Autodesk Inventor part; units mm, degrees
ref_plane "C1_XY" through (0, 0, 0) normal (0, 0, 1) x (1, 0, 0)
ref_plane "C1_YZ" through (0, 0, 0) normal (1, 0, 0) x (0, 1, 0)
ref_plane "C1_ZX" through (0, 0, 0) normal (0, 1, 0) x (0, 0, 1)
sketch "Sketch_1" plane through (0, 0, 0) normal (0, 0, 1) x (1, 0, 0)
  line L0 (-15, -4) -> (-15, -13)
  arc A0 (-15, -13) -> (-13, -15) centre (-13, -13) ccw
  line L1 (-13, -15) -> (-4, -15)
  line L2 (-4, -15) -> (-4, -13)
  line L3 (-4, -13) -> (-8.25, -13)
  line L4 (-8.25, -13) -> (-8.25, -9.6642)
  line L5 (-8.25, -9.6642) -> (-4.5858, -6)
  line L6 (-4.5858, -6) -> (-0.5196, -6)
  line L7 (-0.5196, -6) -> (0, -5.7)
  line L8 (0, -5.7) -> (0.5196, -6)
  line L9 (0.5196, -6) -> (4.5858, -6)
  line L10 (4.5858, -6) -> (8.25, -9.6642)
  line L11 (8.25, -9.6642) -> (8.25, -13)
  line L12 (8.25, -13) -> (4, -13)
  line L13 (4, -13) -> (4, -15)
  line L14 (4, -15) -> (13, -15)
  arc A1 (13, -15) -> (15, -13) centre (13, -13) ccw
  line L15 (15, -13) -> (15, -4)
  line L16 (15, -4) -> (13, -4)
  line L17 (13, -4) -> (13, -8.25)
  line L18 (13, -8.25) -> (9.6642, -8.25)
  line L19 (9.6642, -8.25) -> (6, -4.5858)
  line L20 (6, -4.5858) -> (6, -0.5196)
  line L21 (6, -0.5196) -> (5.7, 0)
  line L22 (5.7, 0) -> (6, 0.5196)
  line L23 (6, 0.5196) -> (6, 4.5858)
  line L24 (6, 4.5858) -> (9.6642, 8.25)
  line L25 (9.6642, 8.25) -> (13, 8.25)
  line L26 (13, 8.25) -> (13, 4)
  line L27 (13, 4) -> (15, 4)
  line L28 (15, 4) -> (15, 13)
  arc A2 (15, 13) -> (13, 15) centre (13, 13) ccw
  line L29 (13, 15) -> (4, 15)
  line L30 (4, 15) -> (4, 13)
  line L31 (4, 13) -> (8.25, 13)
  line L32 (8.25, 13) -> (8.25, 9.6642)
  line L33 (8.25, 9.6642) -> (4.5858, 6)
  line L34 (4.5858, 6) -> (0.5196, 6)
  line L35 (0.5196, 6) -> (0, 5.7)
  line L36 (0, 5.7) -> (-0.5196, 6)
  line L37 (-0.5196, 6) -> (-4.5858, 6)
  line L38 (-4.5858, 6) -> (-8.25, 9.6642)
  line L39 (-8.25, 9.6642) -> (-8.25, 13)
  line L40 (-8.25, 13) -> (-4, 13)
  line L41 (-4, 13) -> (-4, 15)
  line L42 (-4, 15) -> (-13, 15)
  arc A3 (-13, 15) -> (-15, 13) centre (-13, 13) ccw
  line L43 (-15, 13) -> (-15, 4)
  line L44 (-15, 4) -> (-13, 4)
  line L45 (-13, 4) -> (-13, 8.25)
  line L46 (-13, 8.25) -> (-9.6642, 8.25)
  line L47 (-9.6642, 8.25) -> (-6, 4.5858)
  line L48 (-6, 4.5858) -> (-6, 0.5196)
  line L49 (-6, 0.5196) -> (-5.7, 0)
  line L50 (-5.7, 0) -> (-6, -0.5196)
  line L51 (-6, -0.5196) -> (-6, -4.5858)
  line L52 (-6, -4.5858) -> (-9.6642, -8.25)
  line L53 (-9.6642, -8.25) -> (-13, -8.25)
  line L54 (-13, -8.25) -> (-13, -4)
  line L55 (-13, -4) -> (-15, -4)
extrude "Extrusion1" add sketch "Sketch_1" against normal blind 586
sketch "Sketch2" plane through (0, 0, -586) normal (0, 0, -1) x (-1, 0, 0)
  point P0 (0, 0)
hole "Hole1" at (0, 0, -586) direction (0, 0, 1) diameter 6.8 depth 586
sketch "Sketch3" plane through (0, 0, -586) normal (0, 0, -1) x (-1, 0, 0)
  point P0 (-11.6, 11.6)
hole "Hole2" at (11.6, 11.6, -586) direction (0, 0, 1) diameter 4.2 depth 586
pattern_linear "Rectangular Pattern1" count 2 spacing 23.2 along (-1, 0, 0) count 2 spacing 23.2 along (0, -1, 0) of "Hole2"
sketch "Sketch_41" plane through (0, 0, 0) normal (1, 0, 0) x (0, 0, -1)
  line L0 (10, 0) -> (0.05, 0)
  line L1 (0.05, 2.5) -> (0.483, 2.067)
  line L2 (0.483, 2.067) -> (10, 2.067)
  line L3 (10, 2.067) -> (10, 3.45)
  line L4 (10, 3.45) -> (0.05, 3.45)
  line L5 (0.05, 3.45) -> (0.05, 2.5)
revolve "Revolution1" add sketch "Sketch_41" angle 360 about axis through (0, 0, -10) along (0, 0, -1)
thread "Thread1"
sketch "Sketch_42" plane through (0, 0, 0) normal (1, 0, 0) x (0, 0, -1)
  line L0 (585.95, 0) -> (576, 0)
  line L1 (576, 3.45) -> (576, 2.067)
  line L2 (576, 2.067) -> (585.517, 2.067)
  line L3 (585.517, 2.067) -> (585.95, 2.5)
  line L4 (585.95, 2.5) -> (585.95, 3.45)
  line L5 (585.95, 3.45) -> (576, 3.45)
revolve "Revolution2" add sketch "Sketch_42" angle 360 about axis through (0, 0, -585.95) along (0, 0, -1)
thread "Thread2"
ref_plane "C1_XY" through (0, 0, 0) normal (0, 0, 1) x (1, 0, 0)
ref_plane "C1_YZ" through (0, 0, 0) normal (1, 0, 0) x (0, 1, 0)
ref_plane "C1_ZX" through (0, 0, 0) normal (0, 1, 0) x (0, 0, 1)
ref_plane "to_frame_cap1_XY" through (0, 0, 0) normal (0, 0, 1) x (1, 0, 0)
ref_plane "to_frame_cap1_YZ" through (0, 0, 0) normal (1, 0, 0) x (0, 1, 0)
ref_plane "to_frame_cap1_ZX" through (0, 0, 0) normal (0, 1, 0) x (0, 0, 1)
ref_plane "to_frame_cap2_XY" through (0, 0, -586) normal (0, 0, -1) x (1, 0, 0)
ref_plane "to_frame_cap2_YZ" through (0, 0, -586) normal (1, 0, 0) x (0, -1, 0)
ref_plane "to_frame_cap2_ZX" through (0, 0, -586) normal (0, -1, 0) x (0, 0, -1)
properties part number "HFSB6-3030-586-HPW"
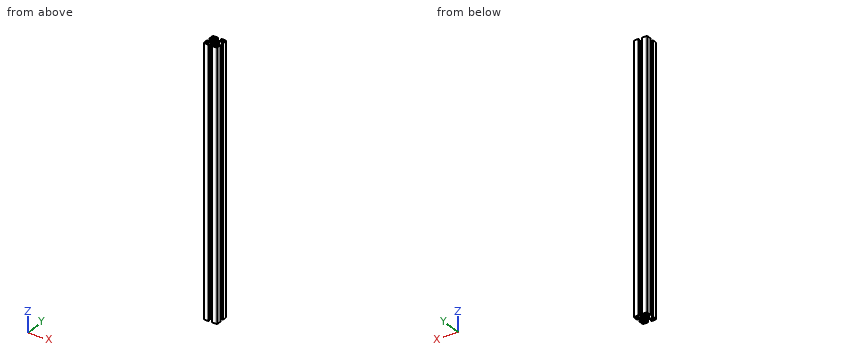
Build history of the part. All positions in model axes, mm. Coordinates: 2 decimals unless noted, no trailing zeros. One line per question, with ' | ' between items. Start each with the question number.
1. Wall check: line 1 along X through (y, z) = (-11.6, -119); line 2 along Y through (x, z) = (11, -297); line 3 along X through (y, z) = (-4.5, -364). Give the ranges that are in metal, low to high. Write a range as [from, to].
2. Cut at A-A (z = -243.5). Count the separate pieces of the cut face and the enclosed holes in it, plus the area to 3 significant figures.
3. Flat gauge pins, fed straight in: P1, Ø2, axis at x = 0, y = 0.5, coming from the +Z side; P2, Ø2, axis at y = 1.5, z = -158, coming from the -X side; P3, Ø6.5, axis at x = 0, y = 0, coming from the -Z side; P4, Ø6, axis at x = -2.5, z = -94.5, coming from the -Y side. Where does each tip first touch, or does it go through?
The answers:
1) line 1: x = [-15, -13.7], [-9.5, -8.25], [8.25, 9.5], [13.7, 15] | line 2: y = [-15, -13.61], [-9.59, -8.25], [8.25, 9.59], [13.61, 15] | line 3: x = [-15, -13], [-6, 6], [13, 15]
2) separate pieces: 1 | enclosed holes: 5 | area: 332 mm2
3) P1: passes through | P2: stops at x = -6 | P3: stops at z = -585.95 | P4: stops at y = -15
